Could you check a few things on this model? Use its own coordinates, in mm. A direction names the side the tool comes from. Give positions to 0.01 mm unless a question says otherwise; leave off trailing zeros. Loops run counter-clockwise (first coordinate to the right, second up) from the corner with the lowest first, then second, coordinate; pieces in that order, holes last. Notation, with made-up numbers: (35.25, -39) - (85.25, -39) arc R15 cw to (85.25, -14) - close; hole circle Ø3 at (7, 64). An arc over 180 degrees is marked (long way). One line per item, written item: value. Start each with the question number.
Q1. If we mould it in two halves opening along Y, with no side actions, what happens to faces 1 (the face through (0, 19.05, -9)), 2 (the face through (0, -21.59, 0)), 3 (the face through (46.985, 0.475, 0.124))? For each: released by +Y, released by -Y, zero draft, split by the parting line, or undercut.
Q2. For faces 4 (the face through (0, 20.32, 0)), 5 (the face through (25.4, 20, -18)), 6 (the face through (0.2, 19.3, 8.89)), 7 (the face through (0, -19.05, 0)), 8 (the face through (-25.4, 20, -18)), which set-ups out of +Z, -Z, +X, -X, +Y, -Y let a thin tool reach every point of the face, with its end or its side?
Q3. If I drill on line 1 (Y direction, x = -11.5, z = 2); line 2 (X direction, y = 0.5, z = 0); line 3 (Y direction, x = -19.5, z = -14), over which ranges is the centre line in solid material (lowest first)? Write a range as from..to.
Q4. I want a section at C-C (z = -1.5). Please give me the cut outline in (x, y), then the cut area to 3 significant figures.
Q5. I'm going to push flat-ended pins straight in: P1, Ø1.5, axis at y = 6, z = 5, coming from the -X side; P2, Ø2, axis at x = 13, z = -11, coming from the -Y side; P3, Ø1.3, axis at y = 20, z = -18, coming from the -X side; P4, Ø1, axis at x = 0, y = 20.5, coming from the +Z side. Where does each tip first touch, or does it pass through?
Q6. I want a section at B-B (x = 21.5). Please give me the cut outline in (y, z), then the cut area to 3 significant figures.
Q7. I want a section at D-D (x = 1). Please give me the cut outline in (y, z), then the cut area to 3 significant figures.
Q8. I want a section at A-A (y = 0). Please give me the cut outline in (x, z).
```python
from build123d import *

# Parameters (mm, degrees)
BOSS_EXTRUDE1_DEPTH            = 8.89
CUT_EXTRUDE1_REACH             = 10.89
SKETCH3_W                      = 7.62
SKETCH3_H                      = 2.54
CUT_EXTRUDE1_DIRECTION_2_REACH = 10.89
SKETCH4_W                      = 50.8
SKETCH4_H                      = 2.54
BOSS_EXTRUDE2_DEPTH            = 17.78


with BuildPart() as part:
    # Sketch2 → Boss-Extrude1 (new body, symmetric)
    with BuildSketch(Plane.XY):
        with BuildLine():
            Line((-25.4, 21.59), (25.4, 21.59))
            ThreePointArc((25.4, 21.59), (46.99, 0), (25.4, -21.59))
            Line((25.4, -21.59), (-25.4, -21.59))
            ThreePointArc((-25.4, -21.59), (-46.99, 0), (-25.4, 21.59))
        make_face()
        with BuildLine():
            Line((-25.4, 19.05), (25.4, 19.05))
            ThreePointArc((25.4, 19.05), (44.45, 0), (25.4, -19.05))
            Line((25.4, -19.05), (-25.4, -19.05))
            ThreePointArc((-25.4, -19.05), (-44.45, 0), (-25.4, 19.05))
        make_face(mode=Mode.SUBTRACT)
    extrude(amount=BOSS_EXTRUDE1_DEPTH, both=True)

    # Sketch3 → Cut-Extrude1 (cut, up to next)
    with BuildSketch(Plane.XY, mode=Mode.PRIVATE) as cut_extrude1_sk1:
        with Locations((0, 21.59)):
            Rectangle(SKETCH3_W, SKETCH3_H)
    cut_extrude1_tool1 = extrude(cut_extrude1_sk1.sketch, amount=-CUT_EXTRUDE1_REACH, mode=Mode.PRIVATE) & part.part
    add(cut_extrude1_tool1.solids().sort_by_distance((0, 21.59, 0))[0], mode=Mode.SUBTRACT)

    # Sketch3 → Cut-Extrude1 direction 2 (cut, up to next)
    with BuildSketch(Plane.XY, mode=Mode.PRIVATE) as cut_extrude1_direction_2_sk1:
        with Locations((0, 21.59)):
            Rectangle(SKETCH3_W, SKETCH3_H)
    cut_extrude1_direction_2_tool1 = extrude(cut_extrude1_direction_2_sk1.sketch, amount=CUT_EXTRUDE1_DIRECTION_2_REACH, mode=Mode.PRIVATE) & part.part
    add(cut_extrude1_direction_2_tool1.solids().sort_by_distance((0, 21.59, 0))[0], mode=Mode.SUBTRACT)

    # Sketch4 → Boss-Extrude2 (add)
    with BuildSketch(Plane(origin=(0, 0, -8.89), x_dir=(-1, 0, 0), z_dir=(0, 0, -1))):
        with Locations((0, 20.32)):
            Rectangle(SKETCH4_W, SKETCH4_H)
    extrude(amount=BOSS_EXTRUDE2_DEPTH)


solid = part.part
```
Worked answers:
1. face 1: undercut
1. face 2: released by -Y
1. face 3: split by the parting line
2. face 4: +Z, +Y
2. face 5: -Z, +X, +Y, -Y
2. face 6: +Z, +X, -X, +Y, -Y
2. face 7: +Z, -Z
2. face 8: -Z, -X, +Y, -Y
3. line 1: y = -21.59..-19.05, 19.05..21.59
3. line 2: x = -46.98..-44.44, 44.44..46.98
3. line 3: y = 19.05..21.59
4. outline: (-25.4, -21.59) - (25.4, -21.59) arc R21.59 ccw to (25.4, 21.59) - (3.81, 21.59) - (3.81, 20.32) - (-3.81, 20.32) - (-3.81, 21.59) - (-25.4, 21.59) arc R21.59 ccw to start; hole (-25.4, -19.05) - (25.4, -19.05) arc R19.05 ccw to (25.4, 19.05) - (-25.4, 19.05) arc R19.05 ccw to start
4. area: 573 mm²
5. P1: stops at x = -46.34
5. P2: stops at y = 19.05
5. P3: stops at x = -25.4
5. P4: stops at z = 8.89
6. outline: (-21.59, -8.89) - (-19.05, -8.89) - (-19.05, 8.89) - (-21.59, 8.89) - close; (19.05, -26.67) - (21.59, -26.67) - (21.59, 8.89) - (19.05, 8.89) - close
6. area: 135 mm²
7. outline: (-21.59, -8.89) - (-19.05, -8.89) - (-19.05, 8.89) - (-21.59, 8.89) - close; (19.05, -26.67) - (21.59, -26.67) - (21.59, -8.89) - (20.32, -8.89) - (20.32, 8.89) - (19.05, 8.89) - close
7. area: 113 mm²
8. outline: (-46.99, -8.89) - (-44.45, -8.89) - (-44.45, 8.89) - (-46.99, 8.89) - close; (44.45, -8.89) - (46.99, -8.89) - (46.99, 8.89) - (44.45, 8.89) - close
